Read the model definition and answer for the solid it produces. Units are mm, in the model's axes. A direction names the side the tool comes from. Coordinates: 2 decimals unless noted, no trailing zeros. Write each loop counter-clockwise with the first axis right and the second up, starting at its lowest first coordinate (ties: lowest second). Pieces come first, ordered by that corner, then holes.
(1) Find the intervals of material crossed by probe 1 along Y at (x, z) = (0, 9.75); probe 2 along Z at (x, y) = (8, -7.75); probe 3 along Y at (x, z) = (-1.5, 15.5), in increasing order.
(2) Which of the six approach directions +Z, -Z, +X, -X, +Y, -Y give full straight-line access (tool end or side, diameter ignored) to faces 1 (the cylindrical face through (11.207, -3.529, 11.092)), 2 (the flat face through (5, -2, 25)), 3 (the flat face through (0, 12, 0))?
(3) The mould has two halves that part along Z. Classify faces 4 (the flat face through (0, 0, 55)), 5 (the cylindrical face through (-1.08, -4.88, 37.33)), 6 (the flat face through (0, 0, 22.5)): +Z half, -Z half, draft (parallel to the pull), parting line (faces both ways), or undercut.
(4) Section C-C on z = 42.5 is taken. Write down the section's boundary in (x, y), then the cut area to 3 significant figures.
(5) Given pin 1 (4 mm diameter, centred on x = -11, y = -2, fed in from +Z); pin 2 (3 mm diameter, centred on x = 6.5, z = 21.5, fed in from +Y); pin 3 (12 mm diameter, centred on x = 9, z = 13.5, fed in from -Y), each flat-ended and moving along its own axis, determine where each tip first touches the part or whether it passes through.
from build123d import *

# Parameters (mm, degrees)
F0_R     = 14.5
F1_DEPTH = 25
F2_R     = 5
F3_DEPTH = 25
F4_R     = 7.5
F5_DEPTH = 5
F6_R     = 2.49999
F7_R     = 3
F8_R     = 11.75
F9_DEPTH = 22.5


# Not quite as in the source:
# - a fillet or chamfer is up to 0.001 mm smaller than in the source, because OpenCascade refuses the exact size


with BuildPart() as f1:
    # F0 (on Top) → F1 (new body)
    with BuildSketch(Plane.XY):
        Circle(F0_R)
    extrude(amount=F1_DEPTH)

    # F2 (on face) → F3 (join)
    with BuildSketch(Plane.XY.offset(25)):
        Circle(F2_R)
    extrude(amount=F3_DEPTH)

    # F4 (on face) → F5 (join)
    with BuildSketch(Plane.XY.offset(50)):
        Circle(F4_R)
    extrude(amount=F5_DEPTH)

    # F6 (radius 2.5 in the source; OpenCascade refuses exactly that, so slightly less here)
    f6_edges = [f1.edges().sort_by_distance(p)[0] for p in [
        (-7.5, 0, 50),
        (-7.5, 0, 55),
    ]]
    fillet(f6_edges, radius=F6_R)

    # F7
    f7_edges = [f1.edges().sort_by_distance(p)[0] for p in [
        (-14.5, 0, 25),
    ]]
    fillet(f7_edges, radius=F7_R)

    # F8 (on face) → F9 (cut)
    with BuildSketch(Plane(origin=(0, 0, 0), x_dir=(1, 0, 0), z_dir=(0, 0, -1))):
        Circle(F8_R)
    extrude(amount=-F9_DEPTH, mode=Mode.SUBTRACT)


solid = f1.part
Response:
1. probe 1: y = -14.5 to -11.75, 11.75 to 14.5
1. probe 2: z = 22.5 to 25
1. probe 3: y = -14.42 to -11.65, 11.65 to 14.42
2. face 1: -Z
2. face 2: none
2. face 3: -Z, +X, -X, +Y, -Y
3. face 4: +Z half
3. face 5: undercut
3. face 6: -Z half
4. outline: circle Ø10 at (0, 0)
4. area: 78.5 mm2
5. pin 1: stops at z = 25
5. pin 2: stops at y = 13.61
5. pin 3: stops at y = -14.19
